from build123d import *

# Parameters (mm, degrees)
SKETCH002_W = 8.5
SKETCH002_H = 2.9
SKETCH003_W = 8.5
SKETCH003_H = 2.9


with BuildPart() as part:
    # Sketch001 → AdditiveLoft section 0
    with BuildSketch(Plane.XY.offset(6.9)):
        with BuildLine():
            Line((-11.9, -5.4), (11.9, -5.4))
            Line((11.9, -5.4), (11.9, -3.8))
            Line((11.9, -3.8), (13.65, -3.8))
            Line((13.65, -3.8), (13.65, -1.9))
            ThreePointArc((11.75, 0), (12.306497, -1.343503), (13.65, -1.9))
            Line((-11.75, 0), (11.75, 0))
            ThreePointArc((-13.65, -1.9), (-12.306497, -1.343503), (-11.75, 0))
            Line((-13.65, -3.8), (-13.65, -1.9))
            Line((-11.9, -3.8), (-13.65, -3.8))
            Line((-11.9, -5.4), (-11.9, -3.8))
        make_face()
    # Sketch → AdditiveLoft section 1
    with BuildSketch(Plane.XY):
        with BuildLine():
            Line((-11.6, -5.4), (11.6, -5.4))
            Line((11.6, -5.4), (11.6, -3.8))
            Line((11.6, -3.8), (13.65, -3.8))
            Line((13.65, -3.8), (13.65, -1.9))
            ThreePointArc((11.75, 0), (12.306497, -1.343503), (13.65, -1.9))
            Line((-11.75, 0), (11.75, 0))
            ThreePointArc((-13.65, -1.9), (-12.306497, -1.343503), (-11.75, 0))
            Line((-13.65, -3.8), (-13.65, -1.9))
            Line((-11.6, -3.8), (-13.65, -3.8))
            Line((-11.6, -5.4), (-11.6, -3.8))
        make_face()
    loft()

    # Sketch002 → SubtractiveLoft section 0
    with BuildSketch(Plane.XZ):
        with Locations((-6.25, 5.45)):
            Rectangle(SKETCH002_W, SKETCH002_H)
    # Sketch003 → SubtractiveLoft section 1
    with BuildSketch(Plane.XZ.offset(5.4)):
        with Locations((-6.25, 5.45)):
            Rectangle(SKETCH003_W, SKETCH003_H)
    loft(mode=Mode.SUBTRACT)


solid = part.part
Could you check a few things on this model? Use its own coordinates, in mm. A direction names the side the tool comes from. Round coordinates to 2 decimals unless told otherwise and drop trailing zeros. Order: outer loops, then holes, each group sorted by start corner. A loop starts at its lowest first (then second) coordinate and runs counter-clockwise, first axis right, second up.
(1) I'm going to push a flat-ended pin straight in: pin 1 (2 mm diameter, centred on x = -11, z = 2.5, fed in from +Y). Where does the tip first touch, or does it pass through?
Response values:
pin 1: stops at y = 0
(2) Imagine slicing it at A-A (y = -2.9). Write out the boundary of the cut face in (x, z).
Response values:
outline: (-13.65, 0) - (13.65, 0) - (13.65, 6.9) - (-2, 6.9) - (-2, 4) - (-10.5, 4) - (-10.5, 6.9) - (-13.65, 6.9) - close
(3) If we mould it in two halves opening along X, with no side actions, what happens to faces 4 (the flat face through (-2, -3, 5)), 5 (the flat face through (13.65, -3, 3)), 6 (the flat face through (3, 0, 3)), 7 (the flat face through (-10.5, -3, 5))? For each: released by +X, released by -X, zero draft, split by the parting line, or undercut.
Response values:
face 4: undercut
face 5: released by +X
face 6: zero draft
face 7: undercut
(4) Please list where these lines run through material, in increasing order: line 1 along Z through (x, y) = (-4.5, -4.5); line 2 along X through (y, z) = (-3.95, 6.25); line 3 along X through (y, z) = (-1.6, 6.75).
Response values:
line 1: z = 0 to 4
line 2: x = -11.87 to -10.5, -2 to 11.87
line 3: x = -12.63 to -10.5, -2 to 12.63
(5) Which directions (+Z, -Z, +X, -X, +Y, -Y) give clear straight access to the entire face, cutting with the end or side of a thin tool? Please do faces 1 (the flat face through (11.748, -4.611, 3.402)), 2 (the flat face through (-11.748, -4.589, 3.402)), 3 (the flat face through (-6, -3, 4)).
Response values:
face 1: -Z, +X, -Y
face 2: -Z, -X, -Y
face 3: +Z, +Y, -Y
(6) Imagine slicing it at B-B (y = -4.5). Write out the boundary of the cut face in (x, z), plus the area to 4 significant figures.
Response values:
outline: (-11.9, 6.9) - (-11.6, 0) - (11.6, 0) - (11.9, 6.9) - (-2, 6.9) - (-2, 4) - (-10.5, 4) - (-10.5, 6.9) - close
area: 137.5 mm2
